Build history of the part. All positions in model axes, mm. Face numbers are marked on the shaded views. A direction names the side the tool comes from. Round coordinates to 2 decimals unless told otherwise and drop trailing zeros. Order: outer loops, then holes, each group sorted by start corner. A loop starts at its lowest first (then second) coordinate and runs counter-clockwise, first axis right, second up. Notation, with made-up numbers: (13.5, 79.25) - (41.5, 79.25) arc R35 ccw to (41.5, 112.25) - close; hole circle Ø1 at (24, 56). An arc over 180 degrees is marked (long way). One line per question, with ' | ' between items. Start each with the question number.
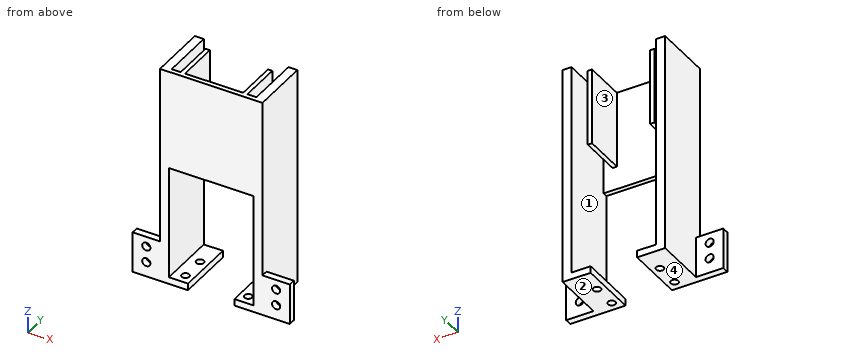
from build123d import *

# Parameters (mm, degrees)
SKETCH1_R             = 2.75
BOSS_EXTRUDE1_DEPTH   = 5
BOSS_EXTRUDE1_2_DEPTH = 5
SKETCH16_W            = 6.5
SKETCH16_H            = 43
BOSS_EXTRUDE2_DEPTH   = 162.9
SKETCH18_W            = 80
SKETCH18_H            = 3.5
BOSS_EXTRUDE3_DEPTH   = 64.9
SKETCH19_W            = 5
SKETCH19_H            = 39.5
BOSS_EXTRUDE4_DEPTH   = 64.9
SKETCH20_W            = 30
SKETCH20_H            = 5
BOSS_EXTRUDE5_DEPTH   = 20
SKETCH21_W            = 30
SKETCH21_H            = 5
BOSS_EXTRUDE6_DEPTH   = 20
SKETCH22_R            = 3
CUT_EXTRUDE1_DEPTH    = 20
SKETCH24_W            = 3.140120034
SKETCH24_H            = 30.638672015
SKETCH24_W_2          = 3.14
BOSS_EXTRUDE8_DEPTH   = 58
SKETCH25_W            = 75
SKETCH25_H            = 43
CUT_EXTRUDE2_DEPTH    = 7


with BuildPart() as part:
    # Sketch1 → Boss-Extrude1 (new body)
    with BuildSketch(Plane.XY):
        Polygon((20.5, 43), (20.5, 18), (20.5, 0), (0, 0), (0, 43), align=None)
        with Locations((14.5, 25)):
            Circle(SKETCH1_R, mode=Mode.SUBTRACT)
        with Locations((14.5, 7)):
            Circle(SKETCH1_R, mode=Mode.SUBTRACT)
    extrude(amount=BOSS_EXTRUDE1_DEPTH)



with BuildPart() as body_2:
    # Sketch1 → Boss-Extrude1 2 (new body)
    with BuildSketch(Plane.XY):
        Polygon((75, 0), (75, 43), (54.5, 43), (54.5, 18), (54.5, 0), align=None)
        with Locations((60.5, 7)):
            Circle(SKETCH1_R, mode=Mode.SUBTRACT)
        with Locations((60.5, 25)):
            Circle(SKETCH1_R, mode=Mode.SUBTRACT)
    extrude(amount=BOSS_EXTRUDE1_2_DEPTH)


with BuildPart() as part_1:
    add(part.part)

    add(body_2.part)  # Boss-Extrude2 merges body 2
    # Sketch16 → Boss-Extrude2 (add)
    with BuildSketch(Plane.XY.offset(5)):
        with Locations((71.75, 21.5)):
            Rectangle(SKETCH16_W, SKETCH16_H)
        with Locations((3.25, 21.5)):
            Rectangle(SKETCH16_W, SKETCH16_H)
    extrude(amount=BOSS_EXTRUDE2_DEPTH)

    # Sketch18 → Boss-Extrude3 (add)
    with BuildSketch(Plane.ZY.offset(-68.5)):
        with Locations((127.9, 1.75)):
            Rectangle(SKETCH18_W, SKETCH18_H)
    extrude(amount=BOSS_EXTRUDE3_DEPTH)

    # Sketch19 → Boss-Extrude4 (add)
    with BuildSketch(Plane.ZY.offset(-68.5)):
        with Locations((165.4, 23.25)):
            Rectangle(SKETCH19_W, SKETCH19_H)
    extrude(amount=BOSS_EXTRUDE4_DEPTH)

    # Sketch20 → Boss-Extrude5 (add)
    with BuildSketch(Plane.ZY):
        with Locations((15, 2.5)):
            Rectangle(SKETCH20_W, SKETCH20_H)
    extrude(amount=BOSS_EXTRUDE5_DEPTH)

    # Sketch21 → Boss-Extrude6 (add)
    with BuildSketch(Plane(origin=(75, 0, 0), x_dir=(0, 0, -1), z_dir=(1, 0, 0))):
        with Locations((-15, 2.5)):
            Rectangle(SKETCH21_W, SKETCH21_H)
    extrude(amount=BOSS_EXTRUDE6_DEPTH)

    # Sketch22 → Cut-Extrude1 (cut)
    with BuildSketch(Plane(origin=(0, 5, 0), x_dir=(1, 0, 0), z_dir=(0, 1, 0))):
        with Locations(Location((-10, -10.799084074, 0), (0, 0, 270))):
            Circle(SKETCH22_R)
        with Locations(Location((-10, -22.633830435, 0), (0, 0, 270))):
            Circle(SKETCH22_R)
        with Locations(Location((85, -10.799084074, 0), (0, 0, 270))):
            Circle(SKETCH22_R)
        with Locations(Location((85, -22.633830435, 0), (0, 0, 270))):
            Circle(SKETCH22_R)
    extrude(amount=-CUT_EXTRUDE1_DEPTH, mode=Mode.SUBTRACT)

    # Sketch24 → Boss-Extrude8 (add)
    with BuildSketch(Plane(origin=(0, 0, 162.9), x_dir=(-1, 0, 0), z_dir=(0, 0, -1))):
        with Locations((-60.320060017, 18.819336008)):
            Rectangle(SKETCH24_W, SKETCH24_H)
        with Locations((-14.68, 18.819336008)):
            Rectangle(SKETCH24_W_2, SKETCH24_H)
    extrude(amount=BOSS_EXTRUDE8_DEPTH)

    # Sketch25 → Cut-Extrude2 (cut)
    with BuildSketch(Plane.XY.offset(167.9)):
        with Locations((37.5, 21.5)):
            Rectangle(SKETCH25_W, SKETCH25_H)
    extrude(amount=-CUT_EXTRUDE2_DEPTH, mode=Mode.SUBTRACT)


solid = part_1.part
Item 1: Slice it at B-B (y = 38). Write the cut outline in (x, z), plus the area to 3 significant figures.
Item 2: Slice it at C-C (z = 33.5). Write the cut outline in (x, y), plus the area to 3 significant figures.
Item 3: Slice it at D-D (x = 85). Write the cut outline in (y, z).
Item 4: 3-axis set-ups, long thin cutter, end or side, ignore diameter. For the marked faces 3 and 4: which of +Z, -Z, +X, -X, +Y, -Y reach the whole face in a straight line?
Item 5: Wall check: line 1 along X through (y, z) = (19, 116); line 2 along X through (y, z) = (36, 72.5); line 3 along Y through (x, z) = (14, 2). Give the ranges that are in metal, low to high. Write a range as [from, to].
Item 6: Slice it at A-A (y = 7). Write the cut outline in (x, z).
Item 7: Pull direction X, two halves, no side cores. Call the marked faces 1 and 2: released by +X, released by -X, zero draft, split by the parting line, or undercut.
Item 8: Pin check, flat tips, straight feed: pin 1 (3.5 mm diameter, centred on x = 60.5, y = 7, fed in from -Z); pin 2 (9 mm diameter, centred on y = 22.5, z = 141.5, fed in from +X); pin 3 (11 mm diameter, centred on x = 12.5, y = 13.5, fed in from +Z); pin 4 (1.5 mm diameter, centred on x = 15.5, y = 35.5, fed in from +Z). Stop position of each tip, or through.
A:
1) outline: (0, 0) - (20.5, 0) - (20.5, 5) - (6.5, 5) - (6.5, 160.9) - (0, 160.9) - close; (54.5, 0) - (75, 0) - (75, 160.9) - (68.5, 160.9) - (68.5, 5) - (54.5, 5) - close | area: 2,230 mm^2
2) outline: (0, 0) - (6.5, 0) - (6.5, 43) - (0, 43) - close; (68.5, 0) - (75, 0) - (75, 43) - (68.5, 43) - close | area: 559 mm^2
3) outline: (0, 0) - (5, 0) - (5, 7.8) - (0, 7.8) - close; (0, 13.8) - (5, 13.8) - (5, 19.63) - (0, 19.63) - close; (0, 25.63) - (5, 25.63) - (5, 30) - (0, 30) - close
4) face 3: +Z, +Y | face 4: -Z, +X, -X, +Y, -Y
5) line 1: [0, 6.5], [13.11, 16.25], [58.75, 61.89], [68.5, 75] | line 2: [0, 6.5], [68.5, 75] | line 3: [0, 4.3], [9.7, 22.3], [27.7, 43]
6) outline: (0, 0) - (11.75, 0) - (11.75, 5) - (6.5, 5) - (6.5, 160.9) - (0, 160.9) - close; (13.11, 104.9) - (16.25, 104.9) - (16.25, 160.9) - (13.11, 160.9) - close; (17.25, 0) - (20.5, 0) - (20.5, 5) - (17.25, 5) - close; (54.5, 0) - (57.75, 0) - (57.75, 5) - (54.5, 5) - close; (58.75, 104.9) - (61.89, 104.9) - (61.89, 160.9) - (58.75, 160.9) - close; (63.25, 0) - (75, 0) - (75, 160.9) - (68.5, 160.9) - (68.5, 5) - (63.25, 5) - close
7) face 1: undercut | face 2: zero draft
8) pin 1: z = 104.9 | pin 2: x = 75 | pin 3: z = 160.9 | pin 4: z = 5
